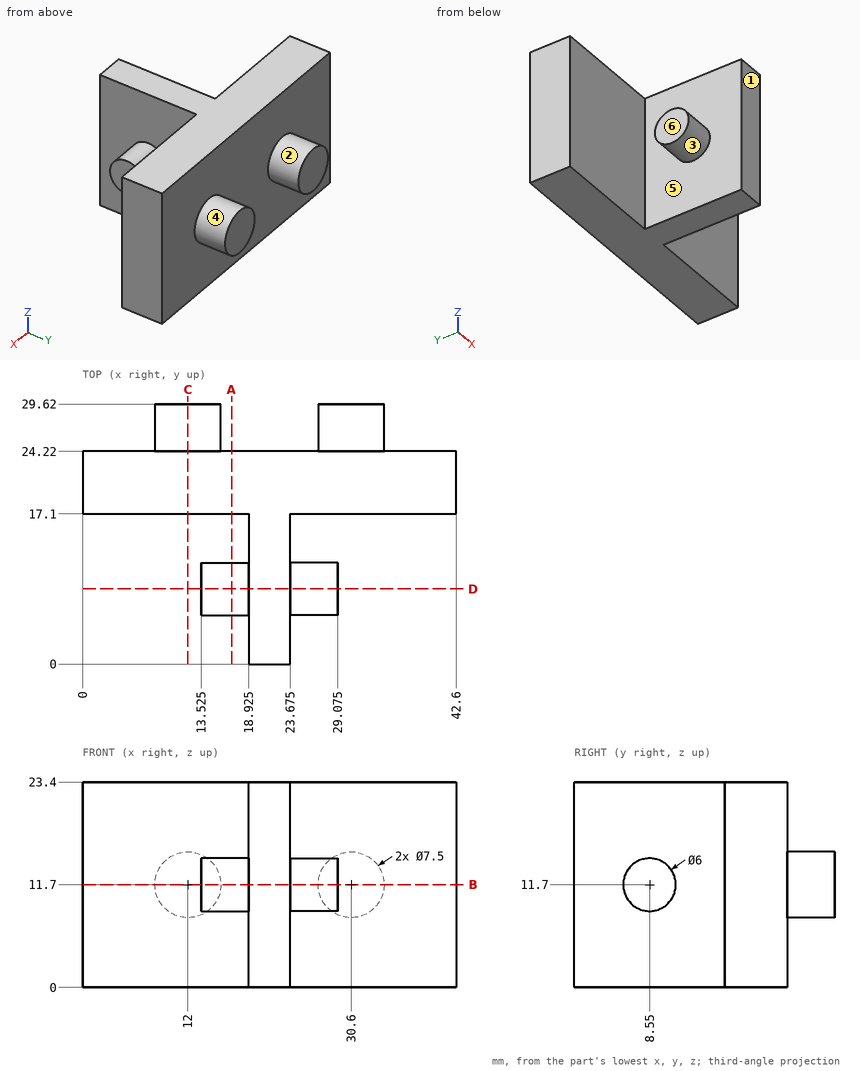
The drawing under review shows one solid part. Ordinate dimensions are in mm from its lowest x, y, z. A direction names the side the tool comes from. Coordinates: 2 decimals unless noted, no trailing zeros. Order: outer loops, then holes, each group sorted by start corner. A loop starts at its lowest first (then second) coordinate and runs counter-clockwise, first axis right, second up. Notation, with made-up numbers: (-14.75, 52.5) -> (20.25, 52.5) arc R29 cw to (20.25, 84.5) -> close; hole circle Ø1 at (11, -26). An arc over 180 degrees is marked (long way). Use CSV: the item, a comma, the result in double quotes. Start each with the question number.
Item 1: We need section D-D, the plane y = 8.55. Give the boundary of the cut face in (x, z) (3 decimals).
Item 2: Insertion check: pin 1 (1.5 mm diameter, centred on y = 20.5, z = 19, fed in from -X); pin 2 (9.5 mm diameter, centred on x = 30.5, z = 12, fed in from -Y); pin 3 (6.5 mm diameter, centred on y = 9, z = 12, fed in from +X) (3 decimals); pin 4 (1.8 mm diameter, centred on y = 9, z = 10.5, fed in from -X) (3 decimals). Each pin has a flat end and moves straight along its axis. Give the tip position at first contact, or say it passes through.
Item 3: We need section B-B, the plane z = 11.7. Give the boundary of the cut face in (x, y) (3 decimals).
Item 4: For the marked faces 4, 5 and 6, list the 3-axis set-ups (+Z, -Z, +X, -X, +Y, -Y) from which the entire face can be reached by the end or side of a thin tool; tool diameter is ignored.
Item 5: Wall thickness on probe 1 along Y at (x, z) = (28.5, 4.5); probe 2 along X at (y, z) = (6, 10.25) (3 decimals); probe 3 along X at (y, z) = (14.25, 5) (3 decimals): over which ranges is each line inside the solid? List them lowest first.
Item 6: Draft analysis for pull direction Y (two halves, no side actions). For the marked faces 1, 2 and 3, state which applies: pulls with the +Y half, pulls with the -Y half, needs draft (parallel to the pull), parting line crosses it, or undercut.
Item 7: We need section C-C, the plane x = 12. Give the boundary of the cut face in (y, z).
Item 8: We need section A-A, the plane x = 17. Give the boundary of the cut face in (y, z), then the cut area to 3 significant figures.
Derived:
1,outline,"(13.525, 8.7) -> (18.925, 8.7) -> (18.925, 0) -> (23.675, 0) -> (23.675, 8.7) -> (29.075, 8.7) -> (29.075, 14.7) -> (23.675, 14.7) -> (23.675, 23.4) -> (18.925, 23.4) -> (18.925, 14.7) -> (13.525, 14.7) -> close"
2,pin 1,"stops at x = 0"
2,pin 2,"stops at y = 5.55"
2,pin 3,"stops at x = 29.075"
2,pin 4,"stops at x = 13.525"
3,outline,"(0, 17.1) -> (18.925, 17.1) -> (18.925, 11.55) -> (13.525, 11.55) -> (13.525, 5.55) -> (18.925, 5.55) -> (18.925, 0) -> (23.675, 0) -> (23.675, 5.55) -> (29.075, 5.55) -> (29.075, 11.55) -> (23.675, 11.55) -> (23.675, 17.1) -> (42.6, 17.1) -> (42.6, 24.22) -> (34.35, 24.22) -> (34.35, 29.62) -> (26.85, 29.62) -> (26.85, 24.22) -> (15.75, 24.22) -> (15.75, 29.62) -> (8.25, 29.62) -> (8.25, 24.22) -> (0, 24.22) -> close"
4,face 4,"+Y"
4,face 5,"-X"
4,face 6,"+Z, -Z, -X, -Y"
5,probe 1,"y = 17.1 to 24.22"
5,probe 2,"x = 13.525 to 29.075"
5,probe 3,"x = 18.925 to 23.675"
6,face 1,"pulls with the -Y half"
6,face 2,"needs draft"
6,face 3,"undercut"
7,outline,"(17.1, 0) -> (24.22, 0) -> (24.22, 7.95) -> (29.62, 7.95) -> (29.62, 15.45) -> (24.22, 15.45) -> (24.22, 23.4) -> (17.1, 23.4) -> close"
8,outline,"circle Ø6 at (8.55, 11.7); (17.1, 0) -> (24.22, 0) -> (24.22, 23.4) -> (17.1, 23.4) -> close"
8,area,"195 mm^2"
